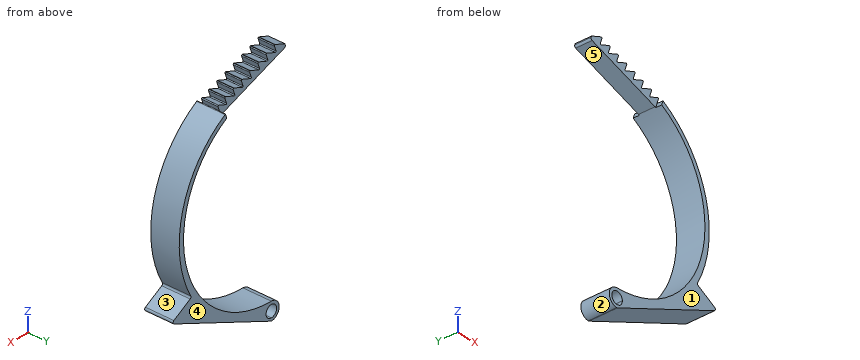
from build123d import *
from build123d.topology import SkipClean

# Parameters (mm, degrees)
BOSS_EXTRUDE1_DEPTH = 13
CUT_EXTRUDE3_DEPTH  = 77.831899265
FILLET1_R           = 0.8
LPATTERN1_DEPTH     = 13
FILLET2_R           = 0.363442
FILLET3_R           = 0.363442
FILLET4_R           = 0.363442
FILLET5_R           = 0.363442
FILLET6_R           = 0.363442
FILLET7_R           = 0.363442
FILLET8_R           = 0.363442
FILLET9_R           = 0.3
SKETCH3_OUTSIDE_W   = 148.316
SKETCH3_OUTSIDE_H   = 39.78
SKETCH3_OUTSIDE_W_2 = 5.910380326
SKETCH3_OUTSIDE_H_2 = 7.5
CUT_EXTRUDE2_DEPTH  = 35.5


# Read off the part's stored shape, not the designer's step: LPattern1
with BuildPart() as part:
    # Sketch1 → Boss-Extrude1 (new body)
    with BuildSketch(Plane(origin=(0, 0, 0), x_dir=(1, 0, 0), z_dir=(0, 1, 0))):
        with BuildLine():
            Line((0, 51.7), (0, 53))
            ThreePointArc((0, 53), (-4, 49), (0, 45))
            ThreePointArc((0, 45), (43.466662183, 11.64685703), (22.5, -38.97114317))
            Line((22.5, -38.97114317), (-10.482378388, -50.975747159))
            Line((-10.482378388, -50.975747159), (-8.772277672, -55.674210263))
            Line((-8.772277672, -55.674210263), (24.536452539, -43.550823925))
            Line((24.536452539, -43.550823925), (23.5, -40.703193978))
            ThreePointArc((23.5, -40.703193978), (45.592051892, -11.596446998), (40.913607467, 24.644050161))
            ThreePointArc((40.913607467, 24.644050161), (24.824872502, 41.52042314), (2.696847486, 48.869563675))
            ThreePointArc((2.696847486, 48.869563675), (-1.954760609, 47.137498735), (0, 51.7))
        make_face()
        with BuildLine():
            Line((51.327605208, 30.606319113), (0, 53))
            Line((0, 53), (0, 51.7))
            ThreePointArc((0, 51.7), (1.909188309, 50.909188309), (2.7, 49))
            ThreePointArc((2.7, 49), (2.699211757, 48.934762792), (2.696847486, 48.869563675))
            ThreePointArc((2.696847486, 48.869563675), (24.824872502, 41.52042314), (40.913607467, 24.644050161))
            Line((40.913607467, 24.644050161), (51.327605208, 30.606319113))
        make_face()
    extrude(amount=BOSS_EXTRUDE1_DEPTH)

    # Sketch2 → Cut-Extrude3 (cut, through all)
    with BuildSketch(Plane(origin=(0, 13, 0), x_dir=(1, 0, 0), z_dir=(0, 1, 0))):
        Polygon((-8.772277672, -55.674210263), (-9.969348173, -52.38528609), (-5.013507189, -54.30612969), align=None)
    extrude(amount=-CUT_EXTRUDE3_DEPTH, mode=Mode.SUBTRACT)

    # Fillet1
    fillet1_edges = [part.edges().sort_by_distance(p)[0] for p in [
        (51.327605208, 6.5, -30.606319113),
        (40.913607467, 6.5, -24.644050161),
        (-10.482378388, 6.5, 50.975747159),
        (0, 6.5, -53),
    ]]
    fillet(fillet1_edges, radius=FILLET1_R)

    # LPattern1 outline → LPattern1 (cut)
    with BuildSketch(Plane(origin=(0, 0, 0), x_dir=(1, 0, 0), z_dir=(0, 1, 0))):
        Polygon((-0.784890395, -52.767039045), (-5.74073138, -50.846195445), (-4.543660878, -54.135119618), align=None)
        Polygon((19.630969381, -41.611651575), (20.828039883, -44.900575748), (24.536452539, -43.550823925), (24.520414883, -43.506760826), align=None)
        Polygon((15.402352588, -43.15074222), (16.59942309, -46.439666393), (20.358193573, -45.07158582), align=None)
        Polygon((11.173735794, -44.689832865), (12.370806296, -47.978757038), (16.129576779, -46.610676465), align=None)
        Polygon((6.945119001, -46.22892351), (8.142189502, -49.517847683), (11.900959986, -48.14976711), align=None)
        Polygon((2.716502207, -47.768014155), (3.913572709, -51.056938328), (7.672343192, -49.688857755), align=None)
        Polygon((-1.512114586, -49.3071048), (-0.315044085, -52.596028973), (3.443726399, -51.2279484), align=None)
    extrude(amount=LPATTERN1_DEPTH, mode=Mode.SUBTRACT)

    # Fillet2
    fillet2_edges = [part.edges().sort_by_distance(p)[0] for p in [
        (-4.543660878, 6.5, 54.135119618),
        (-5.013507189, 6.5, 54.30612969),
    ]]
    fillet(fillet2_edges, radius=FILLET2_R)

    # Fillet3
    fillet3_edges = [part.edges().sort_by_distance(p)[0] for p in [
        (-0.315044085, 6.5, 52.596028973),
        (-0.784890395, 6.5, 52.767039045),
    ]]
    fillet(fillet3_edges, radius=FILLET3_R)

    # Fillet4
    fillet4_edges = [part.edges().sort_by_distance(p)[0] for p in [
        (3.443726399, 6.5, 51.2279484),
        (3.913572709, 6.5, 51.056938328),
    ]]
    fillet(fillet4_edges, radius=FILLET4_R)

    # Fillet5
    fillet5_edges = [part.edges().sort_by_distance(p)[0] for p in [
        (8.142189502, 6.5, 49.517847683),
        (7.672343192, 6.5, 49.688857755),
    ]]
    fillet(fillet5_edges, radius=FILLET5_R)

    # Fillet6
    fillet6_edges = [part.edges().sort_by_distance(p)[0] for p in [
        (11.900959986, 6.5, 48.14976711),
        (12.370806296, 6.5, 47.978757038),
    ]]
    fillet(fillet6_edges, radius=FILLET6_R)

    # Fillet7
    fillet7_edges = [part.edges().sort_by_distance(p)[0] for p in [
        (16.129576779, 6.5, 46.610676465),
        (16.59942309, 6.5, 46.439666393),
    ]]
    fillet(fillet7_edges, radius=FILLET7_R)

    # Fillet8
    fillet8_edges = [part.edges().sort_by_distance(p)[0] for p in [
        (20.828039883, 6.5, 44.900575748),
        (20.358193573, 6.5, 45.07158582),
    ]]
    fillet(fillet8_edges, radius=FILLET8_R)

    # Fillet9
    fillet9_edges = [part.edges().sort_by_distance(p)[0] for p in [
        (6.945119001, 6.5, 46.22892351),
        (11.173735794, 6.5, 44.689832865),
        (-1.512114586, 6.5, 49.3071048),
        (2.716502207, 6.5, 47.768014155),
        (24.520414883, 6.5, 43.506760826),
        (19.630969381, 6.5, 41.611651575),
        (15.402352588, 6.5, 43.15074222),
        (-5.74073138, 6.5, 50.846195445),
        (23.5, 6.5, 40.703193978),
    ]]
    fillet(fillet9_edges, radius=FILLET9_R)

    # Sketch3 outside → Cut-Extrude2 (cut)
    with SkipClean():  # the faces are left unmerged after this step: merging them gives an invalid solid
        with BuildSketch(Plane(origin=(-25.639462386, 0, 9.332001131), x_dir=(0.3420201433256706, 0, 0.9396926207859078), z_dir=(-0.9396926207859078, 0, 0.3420201433256706))):
            with Locations((7.46, 6.5)):
                Rectangle(SKETCH3_OUTSIDE_W, SKETCH3_OUTSIDE_H)
            with Locations((47.141631591, 6.5)):
                Rectangle(SKETCH3_OUTSIDE_W_2, SKETCH3_OUTSIDE_H_2, mode=Mode.SUBTRACT)
        extrude(amount=-CUT_EXTRUDE2_DEPTH, mode=Mode.SUBTRACT)


solid = part.part
The listing builds one solid part. Answer for the finished solid, in the listing's coordinates (mm). Face numbers are marked on the shaded views. A direction names the side the tool comes from. Give positions to 0.01 mm unless a question says otherwise; leave off trailing zeros. Order: outer loops, then holes, each group sorted by start corner. A loop starts at its lowest first (then second) coordinate and runs counter-clockwise, first axis right, second up. Notation, with made-up numbers: (27, -6.75) - (44, -6.75) arc R20 ccw to (44, 15.25) - close; hole circle Ø5 at (-19, 89). An arc over 180 degrees is marked (long way). Use one line per item in the form item = value.
1) Consider probe 1 along Z at (x, y) = (0, 7); probe 2 along Z at (x, y) = (0, 2.5); probe 3 along X at (y, z) = (4.5, -49). Determine where each line is inside the solid, lowest interval first. Write a range as [from, to].
Verdict:
probe_1 = [-52.98, -51.7], [-46.3, -45], [47.16, 49.89]
probe_2 = [-52.98, -51.7], [-46.3, -45]
probe_3 = [-4, -2.7], [2.7, 9.17]
2) Each of these flat-tipped pins is pushed along its axis until it touches: pin 1 (6 mm diameter, centred on y = 3, z = -6, fed in from -X); pin 2 (1 mm diameter, centred on x = 44, y = 8, fed in from -Z); pin 3 (5 mm diameter, centred on y = 8.5, z = 16.5, fed in from -X); pin 4 (5 mm diameter, centred on x = 0, z = -49, fed in from -Y). Where does it stop, or does it pass through?
Verdict:
pin_1 = 44.09
pin_2 = -34.02
pin_3 = 40.79
pin_4 = through
3) Find section C-C on z = -3.5. Determine the outline of the cut face in (x, y).
Verdict:
outline = (44.86, 0) - (47.14, 0) - (47.14, 13) - (44.86, 13) - close
4) For the marked faces 3, 4 and 5, determine the directions among +Z, -Z, +X, -X, +Y, -Y from which every point of the face is accessible in a straight line to the end or side of a thin tool.
Verdict:
face_3 = +X, +Y, -Y
face_4 = +Z, -Z, +X, -X, +Y
face_5 = -X, +Y, -Y
5) Find section B-B on z = 19.5. Determine the outline of the cut face in (x, y).
Verdict:
outline = (40.56, 0) - (42.73, 0) - (42.73, 13) - (40.56, 13) - close
6) Find section A-A on x = 1.5. Determine the outline of the cut face in (y, z) (3 decimals), and give its area (3 significant figures).
Verdict:
outline = (0, -52.346) - (13, -52.346) - (13, -51.245) - (0, -51.245) - close; (0, -46.755) - (13, -46.755) - (13, -44.975) - (0, -44.975) - close; (2.75, 46.615) - (10.25, 46.615) - (10.25, 50.475) - (2.75, 50.475) - close
area = 66.4 mm^2
7) The mould has two halves that part along Z. Classify the marked faces 1 and 2: released by +Z, released by -Z, zero draft, split by the parting line, or undercut.
Verdict:
face_1 = zero draft
face_2 = undercut
